Could you check a few things on this model? Use its own coordinates, in mm. Round coordinates to 2 decimals unless told otherwise and drop trailing zeros. Order: outer loops, then holes, each group sorted by start corner. A loop starts at its lowest first (then second) coordinate and runs counter-clockwise, first axis right, second up. Notation, with made-up numbers: (-27.5, 5.25) - (-5.5, 5.25) arc R20 cw to (-5.5, 22.25) - close; hole circle Ø4 at (3.25, 44.25). An arc over 180 degrees is marked (long way). Return JSON: item names as keys, results as strings. Group by question number.
from build123d import *

# Parameters (mm, degrees)
RESSALTO_EXTRUS_O2_DEPTH      = 25
RESSALTO_EXTRUS_O2_DEPTH_BACK = 5
ESBO_O5_W                     = 4.495494134
ESBO_O5_H                     = 25
ESBO_O6_R                     = 1
CORTE_EXTRUS_O3_DEPTH         = 10
ESBO_O7_R                     = 1
CORTE_EXTRUS_O4_DEPTH         = 10
ESBO_O8_R                     = 3.65
CORTE_EXTRUS_O5_DEPTH         = 10
ESBO_O9_R                     = 1.4
CORTE_EXTRUS_O6_DEPTH         = 10
ESBO_O10_R                    = 1.5
CORTE_EXTRUS_O7_DEPTH         = 10


with BuildPart() as part:
    # Esboço5 → Ressalto-extrusão2 (new, two sides: drawn at the far end of the back side and taken through both)
    with BuildSketch(Plane.XY.offset(5).offset(-RESSALTO_EXTRUS_O2_DEPTH_BACK)):
        with Locations((-50.563178661, 37.985502959)):
            Rectangle(ESBO_O5_W, ESBO_O5_H)
    extrude(amount=RESSALTO_EXTRUS_O2_DEPTH + RESSALTO_EXTRUS_O2_DEPTH_BACK)

    # Esboço6 → Corte-extrusão3 (cut)
    with BuildSketch(Plane.ZY.offset(52.810925728)):
        with Locations((2.5, 46.485502959)):
            Circle(ESBO_O6_R)
    extrude(amount=-CORTE_EXTRUS_O3_DEPTH, mode=Mode.SUBTRACT)

    # Esboço7 → Corte-extrusão4 (cut)
    with BuildSketch(Plane.ZY.offset(52.810925728)):
        with Locations((2.5, 29.485502959)):
            Circle(ESBO_O7_R)
    extrude(amount=-CORTE_EXTRUS_O4_DEPTH, mode=Mode.SUBTRACT)

    # Esboço8 → Corte-extrusão5 (cut)
    with BuildSketch(Plane(origin=(-48.315431594, 0, 0), x_dir=(0, 0, -1), z_dir=(1, 0, 0))):
        with Locations((-17.5, 37.985502959)):
            Circle(ESBO_O8_R)
    extrude(amount=-CORTE_EXTRUS_O5_DEPTH, mode=Mode.SUBTRACT)

    # Esboço9 → Corte-extrusão6 (cut)
    with BuildSketch(Plane.ZY.offset(52.810925728)):
        with Locations((17.5, 46.735502959)):
            Circle(ESBO_O9_R)
    extrude(amount=-CORTE_EXTRUS_O6_DEPTH, mode=Mode.SUBTRACT)

    # Esboço10 → Corte-extrusão7 (cut)
    with BuildSketch(Plane.ZY.offset(52.810925728)):
        with Locations((17.5, 29.235502959)):
            Circle(ESBO_O10_R)
    extrude(amount=-CORTE_EXTRUS_O7_DEPTH, mode=Mode.SUBTRACT)


solid = part.part
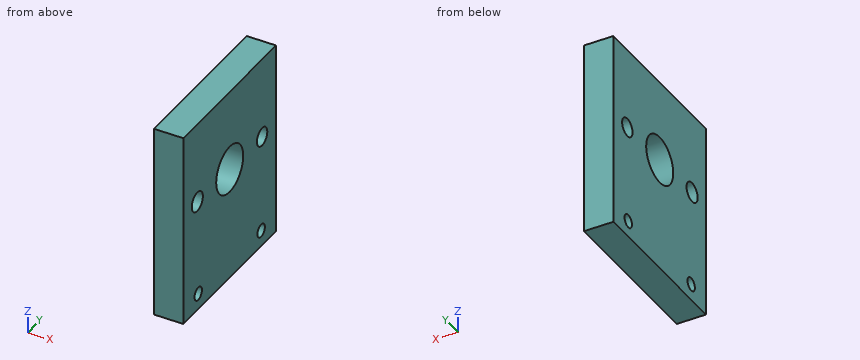
1) I want a section at A-A, the plane z = 2.5. List the corners of the cut face in (x, y) for me, plus the area to 3 significant figures.
2) Will this pin go through, and if not, where does the flat tip stop? pin 1 (1.8 mm diameter, centred on y = 29.24, z = 17.5, fed in from +X).
3) I want a section at D-D, the plane x = -49.75. List the corners of the cut face in (y, z) for me.
4) If I drill on line 1 along Y through (x, z) = (-50.85, 2.5); line 2 along Y through (x, z) = (-50.85, 17.5); line 3 along Z through (x, y) = (-51.2, 38), over which ranges is the centre line in solid material (lowest first)? Write a range as from..to.
5) I want a section at B-B, the plane z = 17.5. List the corners of the cut face in (x, y) for me, plus the area to 3 significant figures.
6) I want a section at C-C, the plane y = 39.25. List the corners of the cut face in (x, z) for me.
Outcome:
{
 "1": {"outline": "(-52.81, 25.49) - (-48.32, 25.49) - (-48.32, 28.49) - (-52.81, 28.49) - close; (-52.81, 30.49) - (-48.32, 30.49) - (-48.32, 45.49) - (-52.81, 45.49) - close; (-52.81, 47.49) - (-48.32, 47.49) - (-48.32, 50.49) - (-52.81, 50.49) - close", "area": "94.4 mm^2"},
 "2": {"pin 1": "through"},
 "3": {"outline": "(25.49, 0) - (50.49, 0) - (50.49, 30) - (25.49, 30) - close; hole circle Ø3 at (29.24, 17.5); hole circle Ø2 at (29.49, 2.5); hole circle Ø7.3 at (37.99, 17.5); hole circle Ø2.8 at (46.74, 17.5); hole circle Ø2 at (46.49, 2.5)"},
 "4": {"line 1": "25.49..28.49, 30.49..45.49, 47.49..50.49", "line 2": "25.49..27.74, 30.74..34.34, 41.64..45.34, 48.14..50.49", "line 3": "0..13.85, 21.15..30"},
 "5": {"outline": "(-52.81, 25.49) - (-48.32, 25.49) - (-48.32, 27.74) - (-52.81, 27.74) - close; (-52.81, 30.74) - (-48.32, 30.74) - (-48.32, 34.34) - (-52.81, 34.34) - close; (-52.81, 41.64) - (-48.32, 41.64) - (-48.32, 45.34) - (-52.81, 45.34) - close; (-52.81, 48.14) - (-48.32, 48.14) - (-48.32, 50.49) - (-52.81, 50.49) - close", "area": "53.5 mm^2"},
 "6": {"outline": "(-52.81, 0) - (-48.32, 0) - (-48.32, 14.08) - (-52.81, 14.08) - close; (-52.81, 20.92) - (-48.32, 20.92) - (-48.32, 30) - (-52.81, 30) - close"}
}
